Check sheet for the modelled part. Datum: model origin and axes. Units: mm. Face numbers are marked on the shaded views. A direction names the side the tool comes from. Give positions to 0.01 mm unless a question says otherwise; leave off trailing zeros. Order: outer loops, then holes, each group sorted by start corner. A loop starts at its lowest first (then second) coordinate and runs counter-clockwise, first axis right, second up. Notation, with made-up numbers: (88, -21.5) - (100, -21.5) arc R31 cw to (100, 12.5) - close; hole circle Ø9 at (-0.75, 17). An arc over 180 degrees is marked (long way). Answer in a Markdown table with one row per item.
Autodesk Inventor part; units mm, degrees
ref_plane "XZ Plane" through (0, 0, 0) normal (0, 1, 0) x (-1, 0, 0)
ref_plane "XY Plane" through (0, 0, 0) normal (0, 0, 1) x (1, 0, 0)
sketch "Skizze1" plane through (0, 0, 0) normal (0, 1, 0) x (-1, 0, 0)
  line L0 (0, 0) -> (7, 0)
  line L1 (7, 0) -> (7, -9)
  line L2 (7, -9) -> (6, -9)
  line L3 (6, -9) -> (6, -114)
  line L4 (6, -114) -> (0, -114)
  line L5 (0, -114) -> (0, 0)
  dimension "d0" = 7
  dimension "d1" = 6
  dimension "d2" = 9
  dimension "d3" = 105
revolve "Umdrehung2" add sketch "Skizze1" angle 360 about axis through (0, 0, -114) along (0, 0, 1)
sketch "Skizze3" plane through (0, 0, -114) normal (0, 0, -1) x (-1, 0, 0)
  point P0 (0, 0)
  point P1 (0, 0)
hole "Bohrung2" at (0, 0, -114) direction (0, 0, 1) diameter 6.647 depth 8 tip angle 118
sketch "Skizze4" plane through (0, 0, 0) normal (0, 0, 1) x (1, 0, 0)
  circle A0 centre (0, 0) radius 3.3235
  point P0 (0, 0)
hole "Bohrung3" at (0, 0, 0) direction (0, 0, -1) diameter 4 end through all
chamfer "Fase2" distance 1 angle 45 1 edges at (0, 2, 0)
ref_plane "Arbeitsebene2" through (6, 0, 0) normal (1, 0, 0) x (0, 1, 0)
sketch "Skizze5" plane through (6, 0, 0) normal (1, 0, 0) x (0, 1, 0)
  line L0 (-6, -114) -> (6, -114)
  line L1 (0, 0) -> (0, -114)
  point P0 (0, -103)
  dimension "d39" = 11
hole "Bohrung4" at (6, 0, -103) direction (-1, 0, 0) diameter 2.459 end up to surface
properties part number "Glashalter"
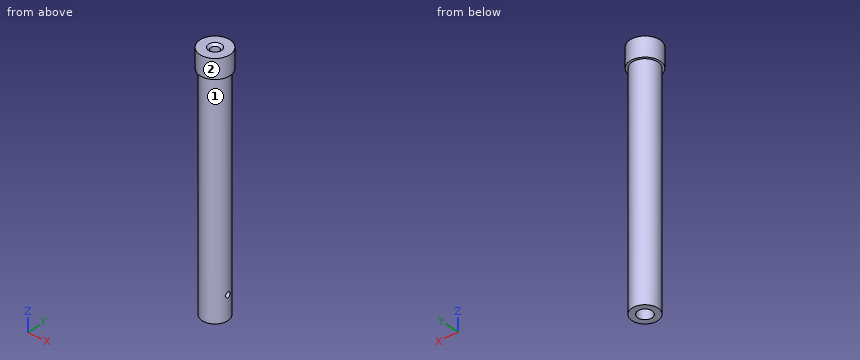
(1) Cross-section at A-A, the plane x = 0. Record the cut outline in (y, z).
Geometry says:
| item | result |
|---|---|
| outline | (-7, -9) - (-6, -9) - (-6, -114) - (-3.32, -114) - (-3.32, -106) - (-2, -105.2) - (-2, -1) - (-3, 0) - (-7, 0) - close; (2, -105.2) - (3.32, -106) - (3.32, -114) - (6, -114) - (6, -9) - (7, -9) - (7, 0) - (3, 0) - (2, -1) - close |
(2) Cross-section at B-B, the plane y = 0. Record the cut outline in (x, z).
Geometry says:
| item | result |
|---|---|
| outline | (-7, -9) - (-6, -9) - (-6, -114) - (-3.32, -114) - (-3.32, -106) - (-2, -105.2) - (-2, -1) - (-3, 0) - (-7, 0) - close; (2, -105.2) - (3.32, -106) - (3.32, -114) - (6, -114) - (6, -104.23) - (2, -104.23) - close; (2, -101.77) - (6, -101.77) - (6, -9) - (7, -9) - (7, 0) - (3, 0) - (2, -1) - close |
(3) Cross-section at C-C, the plane z = -30. Record the cut outline in (x, y).
Geometry says:
| item | result |
|---|---|
| outline | circle Ø12 at (0, 0); hole circle Ø4 at (0, 0) |
(4) Thickness scan on L1, parallel to Y at x = 0, z = -44.5; L2, parallel to X at y = 0, z = -109; L3, parallel to X at y = 0.25, z = -84. Record the ranges inside material, lowest first.
Geometry says:
| item | result |
|---|---|
| L1 | -6 to -2, 2 to 6 |
| L2 | -6 to -3.32, 3.32 to 6 |
| L3 | -5.99 to -1.98, 1.98 to 5.99 |
(5) Cross-section at D-D, the plane x = 5. Record the cut outline in (y, z), then the cut area to 3 significant figures.
Geometry says:
| item | result |
|---|---|
| outline | (-4.9, -9) - (-3.32, -9) - (-3.32, -114) - (3.32, -114) - (3.32, -9) - (4.9, -9) - (4.9, 0) - (-4.9, 0) - close; hole circle Ø2.46 at (0, -103) |
| area | 780 mm² |
(6) Gauge pin test, flat ends, axial feed: P1, Ø5.5, axis at x = 0, y = 0, coming from the +Z side; P2, Ø4, axis at y = -1.5, z = -82.5, coming from the -X side; P3, Ø4.5, axis at x = 0, y = 0, coming from the +Z side. Record the tip position at first contact, or that the pin passes through.
Geometry says:
| item | result |
|---|---|
| P1 | z = -0.25 |
| P2 | x = -6 |
| P3 | z = -0.75 |
(7) Access from +Z, -Z, +X, -X, +Y, -Y to the whole of each face (thin tool, end or side, straight path). Record for the marked faces 1 and 2.
Geometry says:
| item | result |
|---|---|
| face 1 | -Z |
| face 2 | +Z, -Z |
